from build123d import *

# Parameters (mm, degrees)
SKETCH_1_W               = 74.9
SKETCH_1_H               = 74.9
SKETCH_1_W_2             = 66.9
SKETCH_1_H_2             = 66.9
EXTRUDE_1_DEPTH          = 5
SKETCH_2_W               = 85
SKETCH_2_H               = 85
EXTRUDE_2_DEPTH          = 3
FILLET_2_R               = 5
SKETCH_3_W               = 44.125802366
SKETCH_3_H               = 10
CUT_EXTRUDE_1_DEPTH      = 103
PATTERN_CIRCULAR_1_COUNT = 2
PATTERN_CIRCULAR_1_ANGLE = 90
FILLET_3_R               = 2
FILLET_4_R               = 2
FILLET_5_R               = 2
CHAMFER_1_SIZE           = 1
SKETCH_5_R               = 0.8
CUT_EXTRUDE_2_DEPTH      = 10
FILLET_9_R               = 10


with BuildPart() as part:
    # Sketch 1 → Extrude 1 (new body)
    with BuildSketch(Plane(origin=(0, 0, 0), x_dir=(1, 0, 0), z_dir=(0, 1, 0))):
        Rectangle(SKETCH_1_W, SKETCH_1_H)
        Rectangle(SKETCH_1_W_2, SKETCH_1_H_2, mode=Mode.SUBTRACT)
    extrude(amount=EXTRUDE_1_DEPTH)

    # Sketch 2 → Extrude 2 (add)
    with BuildSketch(Plane(origin=(0, 5, 0), x_dir=(1, 0, 0), z_dir=(0, 1, 0))):
        Rectangle(SKETCH_2_W, SKETCH_2_H)
    extrude(amount=EXTRUDE_2_DEPTH)

    # Fillet 2
    fillet_2_edges = [part.edges().sort_by_distance(p)[0] for p in [
        (37.45, 2.5, 37.45),
        (-37.45, 2.5, 37.45),
        (-37.45, 2.5, -37.45),
        (37.45, 2.5, -37.45),
    ]]
    fillet(fillet_2_edges, radius=FILLET_2_R)

    # Sketch 3 → Cut-Extrude 1 (cut, symmetric)
    with BuildSketch(Plane(origin=(0, 0, -37.45), x_dir=(-1, 0, 0), z_dir=(0, 0, -1))):
        Rectangle(SKETCH_3_W, SKETCH_3_H)
    cut_extrude_1 = extrude(amount=CUT_EXTRUDE_1_DEPTH, both=True, mode=Mode.SUBTRACT)

    # Pattern Circular 1: Cut-Extrude 1 ×2 about axis
    pattern_circular_1_axis = Axis((0, 0, 0), (0, -1, 0))
    for i in range(1, PATTERN_CIRCULAR_1_COUNT):
        add(cut_extrude_1.rotate(pattern_circular_1_axis, i * PATTERN_CIRCULAR_1_ANGLE / (PATTERN_CIRCULAR_1_COUNT - 1)), mode=Mode.SUBTRACT)

    # Fillet 3
    fillet_3_edges = [part.edges().sort_by_distance(p)[0] for p in [
        (33.45, 2.5, -33.45),
        (-33.45, 2.5, -33.45),
        (-33.45, 2.5, 33.45),
        (33.45, 2.5, 33.45),
    ]]
    fillet(fillet_3_edges, radius=FILLET_3_R)

    # Fillet 4
    fillet_4_edges = [part.edges().sort_by_distance(p)[0] for p in [
        (-37.45, 2.5, 22.062901183),
        (37.45, 2.5, 22.062901183),
        (-37.45, 2.5, -22.062901183),
        (37.45, 2.5, -22.062901183),
        (22.062901183, 2.5, -37.45),
        (22.062901183, 2.5, 37.45),
        (-22.062901183, 2.5, -37.45),
        (-22.062901183, 2.5, 37.45),
    ]]
    fillet(fillet_4_edges, radius=FILLET_4_R)

    # Fillet 5
    fillet_5_edges = [part.edges().sort_by_distance(p)[0] for p in [
        (-33.45, 5, 26.756450591),
        (33.45, 5, -26.756450591),
        (-26.756450591, 5, 33.45),
        (26.756450591, 5, -33.45),
        (33.45, 5, 26.756450591),
        (-33.45, 5, -26.756450591),
        (-32.864213562, 5, -32.864213562),
        (32.864213562, 5, -32.864213562),
        (32.864213562, 5, 32.864213562),
        (-32.864213562, 5, 32.864213562),
        (-26.756450591, 5, -33.45),
        (26.756450591, 5, 33.45),
    ]]
    fillet(fillet_5_edges, radius=FILLET_5_R)

    # Chamfer 1
    chamfer_1_edges = [part.edges().sort_by_distance(p)[0] for p in [
        (34.45, 0, 22.062901183),
        (-34.45, 0, -22.062901183),
        (-28.256450591, 0, -37.45),
        (-22.062901183, 0, -34.45),
        (-36.864213562, 0, -22.64868762),
        (-22.64868762, 0, -36.864213562),
        (37.45, 0, -28.256450591),
        (34.45, 0, -22.062901183),
        (22.64868762, 0, -36.864213562),
        (36.864213562, 0, -22.64868762),
        (-37.45, 0, 28.256450591),
        (-34.45, 0, 22.062901183),
        (-22.64868762, 0, 36.864213562),
        (-36.864213562, 0, 22.64868762),
        (28.256450591, 0, 37.45),
        (22.062901183, 0, 34.45),
        (22.64868762, 0, 36.864213562),
        (36.864213562, 0, 22.64868762),
        (-28.256450591, 0, 37.45),
        (37.45, 0, 28.256450591),
        (-37.45, 0, -28.256450591),
        (28.256450591, 0, -37.45),
        (35.985533906, 0, 35.985533906),
        (35.985533906, 0, -35.985533906),
        (-35.985533906, 0, -35.985533906),
        (-35.985533906, 0, 35.985533906),
        (22.062901183, 0, -34.45),
        (-22.062901183, 0, 34.45),
    ]]
    chamfer(chamfer_1_edges, length=CHAMFER_1_SIZE)

    # Sketch 5 → Cut-Extrude 2 (cut)
    with BuildSketch(Plane(origin=(0, 5, 0), x_dir=(-1, 0, 0), z_dir=(0, -1, 0))):
        with Locations((-25, 25)):
            Circle(SKETCH_5_R)
        with Locations((25, 25)):
            Circle(SKETCH_5_R)
        with Locations((25, -25)):
            Circle(SKETCH_5_R)
        with Locations((-25, -25)):
            Circle(SKETCH_5_R)
    extrude(amount=-CUT_EXTRUDE_2_DEPTH, mode=Mode.SUBTRACT)

    # Fillet 9
    fillet_9_edges = [part.edges().sort_by_distance(p)[0] for p in [
        (42.5, 6.5, 42.5),
        (42.5, 6.5, -42.5),
        (-42.5, 6.5, -42.5),
        (-42.5, 6.5, 42.5),
    ]]
    fillet(fillet_9_edges, radius=FILLET_9_R)


solid = part.part
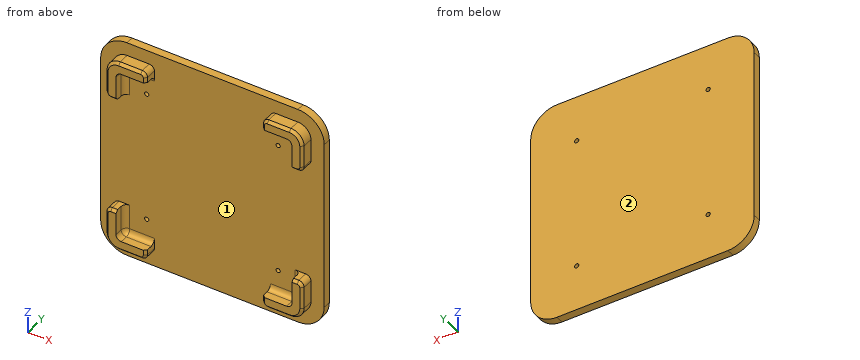
Source: CAD feature listing. Evaluate the final solid. Frame: model axes, mm. Face numbers are marked on the shaded views. Coordinates: 2 decimals unless noted, no trailing zeros. Loops run counter-clockwise (first coordinate to the right, second up) from the corner with the lowest first, then second, coordinate; pieces in that order, holes last. Notation, with made-up numbers: (31, -33.75) -> (45, -33.75) arc R28 ccw to (45, 1.25) -> close; hole circle Ø2 at (86.5, 21.25). An arc over 180 degrees is marked (long way). Answer in a Markdown table with one row per item. Add a question column.
Q1. Section A-A on x = -29.5. Return the cut outline in (y, z).
Q2. Section C-C on x = 4. Return the cut outline in (y, z).
Q3. Section B-B on z = -13.5. Return the cut outline in (x, y).
Q4. Ray query, line 1 along Z through (x, y) = (25, 7.2); line 2 along X through (y, z) = (1, 27). Return the intervals inside material, ascending.
Q5. Pull-direction query (Z, two-part tool) for the marked faces 1 and 2; classes: pulls with the +Z half, pulls with the -Z half, needs draft (parallel to the pull), parting line crosses it, or undercut.
Q6. Contact query for flat-ended pins moving along their axis: pin 1 Ø3.5 at (y, z) = (1, -25.5) entering from +X; pin 2 Ø2 at (y, z) = (2.5, -30) entering from -X; pin 3 Ø0.9 at (x, y) = (-28.5, 1) entering from +Z; pin 4 Ø4.5 at (x, y) = (33, 3.5) entering from +Z. Output: stop coordinate, or through.
Computed values:
| question | item | result |
|---|---|---|
| 1 | outline | (0, -36.45) -> (1, -37.45) -> (5, -37.45) -> (5, -42.5) -> (8, -42.5) -> (8, 42.5) -> (5, 42.5) -> (5, 37.45) -> (1, 37.45) -> (0, 36.45) -> (0, 33.45) -> (3, 33.45) arc R2 cw to (5, 31.45) -> (5, -31.45) arc R2 cw to (3, -33.45) -> (0, -33.45) -> close |
| 2 | outline | (5, -42.5) -> (8, -42.5) -> (8, 42.5) -> (5, 42.5) -> close |
| 3 | outline | (-42.5, 5) -> (42.5, 5) -> (42.5, 8) -> (-42.5, 8) -> close |
| 4 | line 1 | z = -42.5 to -25.8, -24.2 to 24.2, 25.8 to 42.5 |
| 4 | line 2 | x = -37.45 to -33.45, 33.45 to 37.45 |
| 5 | face 1 | undercut |
| 5 | face 2 | needs draft |
| 6 | pin 1 | stops at x = 37.45 |
| 6 | pin 2 | stops at x = -37.45 |
| 6 | pin 3 | stops at z = 37.45 |
| 6 | pin 4 | stops at z = 42.5 |
